Drawing for the job (mm, zero at the part's lowest x, y, z). A direction names the side the tool comes from. Round coordinates to 2 decimals unless told otherwise and drop trailing zeros. Write each loop counter-clockwise with the first axis right and the second up, starting at its lowest first coordinate (ties: lowest second). Pieces come first, ordered by that corner, then holes. Notation, with made-up numbers: (-10.5, 52.5) - (-1.5, 52.5) arc R4 cw to (-1.5, 56.5) - close; hole circle Ø5 at (-8.75, 57.25). An arc over 180 degrees is marked (long way). One line per question, with ' | ' between items.
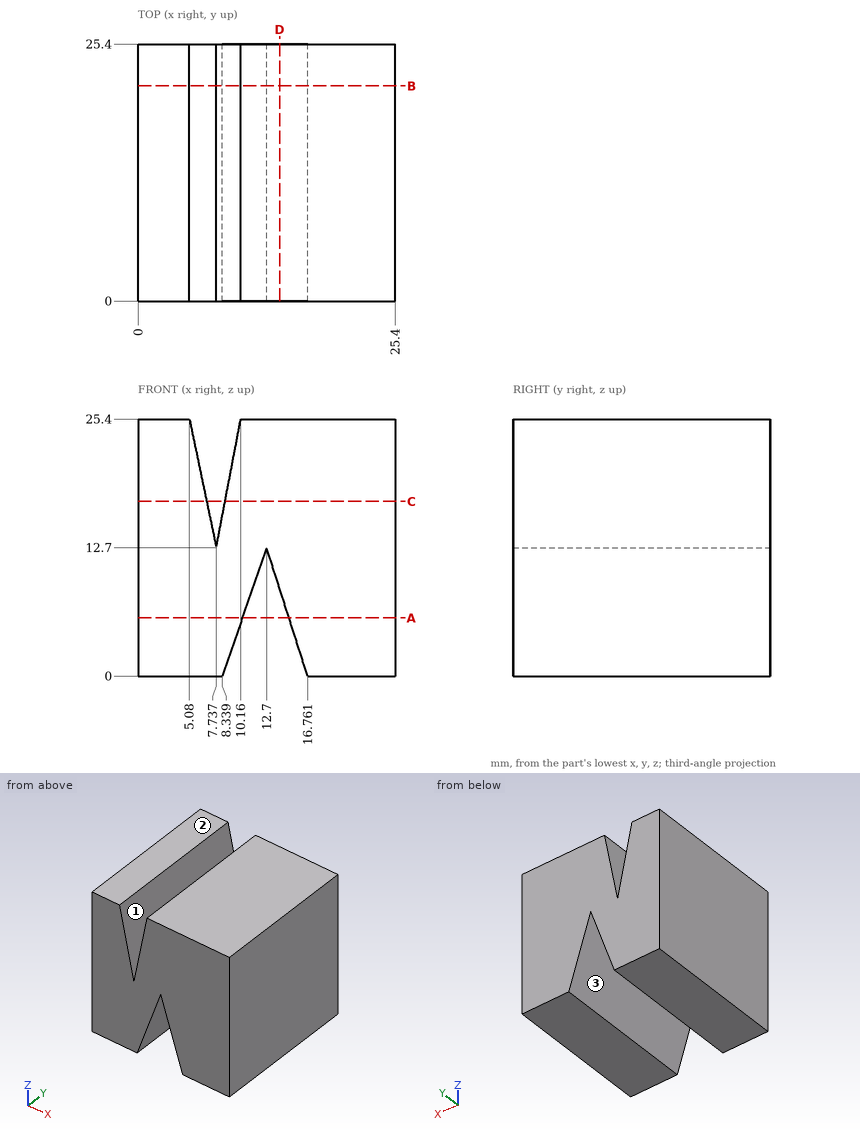
Q1. Saw through at D-D, the plane x = 14. List the corners of the cut face in (y, z) (1 decimal), then the cut area to 3 significant figures.
Found:
outline: (0, 8.6) - (25.4, 8.6) - (25.4, 25.4) - (0, 25.4) - close | area: 426 mm^2
Q2. Saw through at A-A, the plane z = 5.75. List the corners of the cut face in (x, y), then the cut area to 3 significant figures.
Found:
outline: (0, 0) - (10.31, 0) - (10.31, 25.4) - (0, 25.4) - close; (14.92, 0) - (25.4, 0) - (25.4, 25.4) - (14.92, 25.4) - close | area: 528 mm^2
Q3. Which spindle directions (+Z, -Z, +X, -X, +Y, -Y) get a long thin tool onto all of the face, cutting with end or side? Do the marked faces 1, 2 and 3. Say none if no direction does.
Found:
face 1: +Z, +Y, -Y | face 2: +Z, +X, -X, +Y, -Y | face 3: -Z, +Y, -Y
Q4. Saw through at C-C, the plane z = 17.25. List the corners of the cut face in (x, y) (1 decimal), then the cut area to 3 significant figures.
Found:
outline: (0, 0) - (6.8, 0) - (6.8, 25.4) - (0, 25.4) - close; (8.6, 0) - (25.4, 0) - (25.4, 25.4) - (8.6, 25.4) - close | area: 599 mm^2
Q5. Saw through at B-B, the plane y = 21.25. List the corners of the cut face in (x, z).
Found:
outline: (0, 0) - (8.34, 0) - (12.7, 12.7) - (16.76, 0) - (25.4, 0) - (25.4, 25.4) - (10.16, 25.4) - (7.74, 12.7) - (5.08, 25.4) - (0, 25.4) - close
Q6. Drill centre lines: L1, parallel to X at y = 20.5, z = 6.5; L2, parallel to X at y = 8.5, z = 2.5. Where is each one in solid material? Low to high. Write a range as from..to.
Found:
L1: 0..10.57, 14.68..25.4 | L2: 0..9.2, 15.96..25.4
Q7. Drop a flat-ended pin along its axis: pin 1 (2 mm diameter, centred on x = 11.5, z = 22.5, fed in from -Y). Give the stop position or say it passes through.
Found:
pin 1: y = 0
